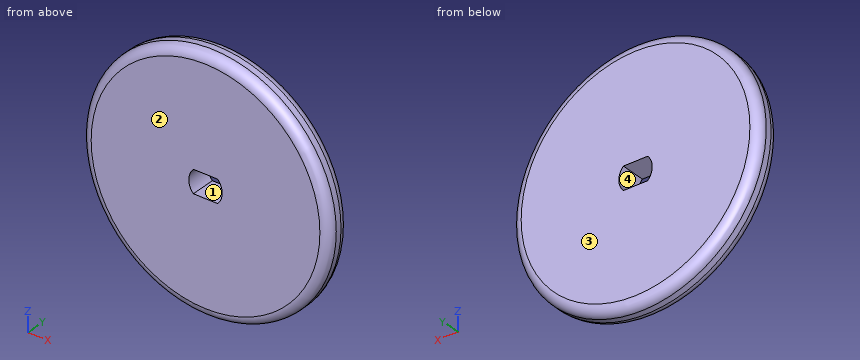
```python
from build123d import *

# Parameters (mm, degrees)
SKETCH_R     = 20
PAD_DEPTH    = 4
FILLET_R     = 1.5
POCKET_DEPTH = 4.001


with BuildPart() as part:
    # Sketch → Pad (new body)
    with BuildSketch(Plane.XZ):
        Circle(SKETCH_R)
    extrude(amount=PAD_DEPTH)

    # Fillet
    fillet_edges = [part.edges().sort_by_distance(p)[0] for p in [
        (-20, -4, 0),
        (-20, 0, 0),
    ]]
    fillet(fillet_edges, radius=FILLET_R)

    # Sketch001 (on Face5 of Fillet) → Pocket (cut, through all)
    with BuildSketch(Plane.XZ.offset(4)):
        with BuildLine():
            ThreePointArc((-1.966596, 1.85), (-2.7, 0), (-1.966596, -1.85))
            Line((-1.966596, -1.85), (1.966596, -1.85))
            ThreePointArc((1.966596, -1.85), (2.7, 0), (1.966596, 1.85))
            Line((-1.966596, 1.85), (1.966596, 1.85))
        make_face()
    extrude(amount=-POCKET_DEPTH, mode=Mode.SUBTRACT)


solid = part.part
```
Verification items for the finished model (mm, model axes). Face numbers are marked on the shaded views. A direction names the side the tool comes from. Give positions to 0.01 mm unless a question says otherwise; leave off trailing zeros. Order: outer loops, then holes, each group sorted by start corner. A loop starts at its lowest first (then second) coordinate and runs counter-clockwise, first axis right, second up. Notation, with made-up numbers: (-10.75, 45) -> (31.25, 45) arc R18 cw to (31.25, 67) -> close; hole circle Ø5 at (29.5, 23). An arc over 180 degrees is marked (long way). Use a Markdown table: item, result.
1) Mould release check, pull along X, two halves, no side actions. Record for the marked faces 1 and 2: pulls with the +X half, pulls with the -X half, needs draft (parallel to the pull), parting line crosses it, or undercut.
Results:
| item | result |
|---|---|
| face 1 | undercut |
| face 2 | needs draft |
2) Material ranges on probe 1 along Z at (x, y) = (-12.5, -0.3); probe 2 along X at (y, z) = (-1.5, 10.5); probe 3 along Z at (x, y) = (16.5, -3.5), recorded low to high.
Results:
| item | result |
|---|---|
| probe 1 | -14.84 to 14.84 |
| probe 2 | -17.02 to 17.02 |
| probe 3 | -10.61 to 10.61 |
3) Tool access check on the marked faces 3 and 4. Record the directions out of +Z, -Z, +X, -X, +Y, -Y that give a thin tool (end or side, any length) a straight path to the whole face; none if there is none.
Results:
| item | result |
|---|---|
| face 3 | +Z, -Z, +X, -X, +Y |
| face 4 | +Y, -Y |
4) Section check A-A, the plane x = 0. Record the boundary of the cut face in (y, z).
Results:
| item | result |
|---|---|
| outline | (-4, -18.5) arc R1.5 ccw to (-2.5, -20) -> (-1.5, -20) arc R1.5 ccw to (0, -18.5) -> (0, -1.85) -> (-4, -1.85) -> close; (-4, 1.85) -> (0, 1.85) -> (0, 18.5) arc R1.5 ccw to (-1.5, 20) -> (-2.5, 20) arc R1.5 ccw to (-4, 18.5) -> close |
5) Section check B-B, the plane z = 0. Record the boundary of the cut face in (x, y).
Results:
| item | result |
|---|---|
| outline | (-20, -2.5) arc R1.5 ccw to (-18.5, -4) -> (-2.7, -4) -> (-2.7, 0) -> (-18.5, 0) arc R1.5 ccw to (-20, -1.5) -> close; (2.7, -4) -> (18.5, -4) arc R1.5 ccw to (20, -2.5) -> (20, -1.5) arc R1.5 ccw to (18.5, 0) -> (2.7, 0) -> close |
6) Section check D-D, the plane y = -3.5. Record the boundary of the cut face in (x, z), then the cut area to 3 significant figures.
Results:
| item | result |
|---|---|
| outline | circle Ø39.24 at (0, 0); hole (-1.97, -1.85) -> (1.97, -1.85) arc R2.7 ccw to (1.97, 1.85) -> (-1.97, 1.85) arc R2.7 ccw to start |
| area | 1,190 mm² |
7) Section check C-C, the plane y = -0.7. Record the boundary of the cut face in (x, z), then the cut area to 3 significant figures.
Results:
| item | result |
|---|---|
| outline | circle Ø39.54 at (0, 0); hole (-1.97, -1.85) -> (1.97, -1.85) arc R2.7 ccw to (1.97, 1.85) -> (-1.97, 1.85) arc R2.7 ccw to start |
| area | 1,210 mm² |
8) Depth check by flat-ended pin: pin 1 Ø2 at (x, y) = (-0.5, -2.5) entering from -Z. Enter the tip coordinate at first touch or a pass-through.
Results:
| item | result |
|---|---|
| pin 1 | z = -20 |
